```python
from build123d import *

# Parameters (mm, degrees)
CHANFREIN1_SIZE         = 0.3
ENL_V_MAT_EXTRU_1_DEPTH = 0.75


with BuildPart() as part:
    # Esquisse1 → Révolution1 (revolve)
    with BuildSketch(Plane.XY, mode=Mode.PRIVATE) as r_volution1_sk:
        Polygon((0, 0), (14, 0), (14, 1.5), (1.7, 1.5), (0.2, 3), (0, 3), align=None)
    revolve(r_volution1_sk.sketch.rotate(Axis((0, 0, 0), (1, 0, 0)), 90), axis=Axis((0, 0, 0), (1, 0, 0)))

    # Chanfrein1
    chanfrein1_edges = [part.edges().sort_by_distance(p)[0] for p in [
        (14, 0, -1.5),
    ]]
    chamfer(chanfrein1_edges, length=CHANFREIN1_SIZE)

    # Esquisse2 → Enlèv. mat.-Extru.1 (cut)
    with BuildSketch(Plane.ZY):
        Polygon((0.577350269, -1), (1.154700538, 0), (0.577350269, 1), (-0.577350269, 1), (-1.154700538, 0), (-0.577350269, -1), align=None)
    extrude(amount=-ENL_V_MAT_EXTRU_1_DEPTH, mode=Mode.SUBTRACT)


solid = part.part
```
Work out the finished part from the listing and answer in its coordinate system (mm). Round coordinates to 2 decimals unless told otherwise and drop trailing zeros. Order: outer loops, then holes, each group sorted by start corner. A loop starts at its lowest first (then second) coordinate and runs counter-clockwise, first axis right, second up.
Q1. Find the intervals of material crossed by line 1 along Z through (x, y) = (1.5, -1.25); line 2 along Y through (x, z) = (11.25, 0.9); line 3 along X through (y, z) = (0.55, -0.7), in increasing order.
Solution:
line 1: z = -1.15 to 1.15
line 2: y = -1.2 to 1.2
line 3: x = 0.75 to 14
Q2. The mould has two halves that part along Y. Classify faces 1 (the flat face through (14, 0, 0)), 2 (the cylindrical face through (7.62, -0.45, 1.43)), 3 (the flat face through (0.75, 0, 0)): pulls with the +Y half, pulls with the -Y half, needs draft (parallel to the pull), parting line crosses it, or undercut.
Solution:
face 1: needs draft
face 2: parting line crosses it
face 3: undercut
Q3. A cutting plane is placed at B-B, the plane x = 7. Determine the outline of the cut face in (y, z), then the cut area to 3 significant figures.
Solution:
outline: circle Ø3 at (0, 0)
area: 7.07 mm2
Q4. A cutting plane is placed at A-A, the plane z = 0. Determine the outline of the cut face in (x, y).
Solution:
outline: (0, -3) - (0.2, -3) - (1.7, -1.5) - (13.7, -1.5) - (14, -1.2) - (14, 1.2) - (13.7, 1.5) - (1.7, 1.5) - (0.2, 3) - (0, 3) - (0, 1) - (0.75, 1) - (0.75, -1) - (0, -1) - close
Q5. Given pin 1 Ø1.5 at (y, z) = (2, -2) entering from -X; pin 2 Ø1.5 at (x, z) = (12, -0.5) entering from +Y; pin 3 Ø0.6 at (y, z) = (0, -0.5) entering from -X; pin 4 Ø1 at (x, y) = (6.5, -2.5) entering from +Z, each flat-ended and moving along its own axis, determine where each tip first touches the part or whether it passes through.
Solution:
pin 1: stops at x = 0
pin 2: stops at y = 1.5
pin 3: stops at x = 0.75
pin 4: passes through
